Autodesk Inventor part; units mm, degrees
ref_plane "Work Plane1" through (29, 0, 0) normal (0, -1, 0) x (1, 0, 0)
ref_plane "YZ Plane" through (0, 0, 0) normal (1, 0, 0) x (0, 1, 0)
ref_plane "XZ Plane" through (0, 0, 0) normal (0, 1, 0) x (-1, 0, 0)
sketch "Sketch1" plane through (0, 0, 0) normal (0, 0, 1) x (1, 0, 0)
  line L0 (-0.9567, 0) -> (11.1125, 0)
  line L1 (11.1125, 0) -> (11.1125, 1.7526)
  line L2 (11.1125, 1.7526) -> (1.9847, 1.7526)
  line L3 (1.9847, 1.7526) -> (0.0001, 1.7526)
  line L4 (0.0001, 1.7526) -> (0, 1.7526)
  line L5 (0, 1.7526) -> (0, 2.8702)
  line L6 (0, 2.8702) -> (-3.5052, 2.8702)
  line L7 (-3.5052, 2.8702) -> (-3.5052, 1.5985)
  line L8 (-3.5052, 1.5985) -> (-1.8796, 1.5985)
  line L9 (-1.8796, 1.5985) -> (-0.9567, 0)
  line L10 (-6.4287, 0) -> (14.036, 0)
  line L11 (0, -0.574) -> (0, 3.4442)
  line L12 (1.9847, 1.7526) -> (0, 1.7526) construction
  dimension "d1" = 9.1278
  dimension "d2" = 1.9846
  dimension "d3" = 3.5052
  dimension "d4" = 1.6256
  dimension "d5" = 60
  dimension "d6" = 3.5052
  dimension "d7" = 3.5052
  dimension "d8" = 3.1969
  dimension "d9" = 5.7404
  dimension "d26" = 11.1125
revolve "Body" add sketch "Sketch1" angle 360 about axis through (-0.9567, 0, 0) along (1, 0, 0)
sketch "Sketch2" plane through (-3.5052, 0, 0) normal (-1, 0, 0) x (0, 0, 1)
  circle A0 centre (0, 0) radius 1.5985
  line L0 (0, -4.0183) -> (0, 4.0183)
  line L1 (-4.0183, 0) -> (4.0183, 0)
  line L2 (1.5985, 0) -> (0.7992, -1.3843)
  line L3 (0.7992, -1.3843) -> (-0.7992, -1.3843)
  line L4 (-0.7992, -1.3843) -> (-1.5985, 0)
  line L5 (-1.5985, 0) -> (-0.7992, 1.3843)
  line L6 (-0.7992, 1.3843) -> (0.7992, 1.3843)
  line L7 (0.7992, 1.3843) -> (1.5985, 0)
extrude "Slot" add sketch "Sketch2" against normal up to next contours L7 A0 | A0 L2 | L6 L0 A0 | A0 L0 L3 | L0 L6 A0 | A0 L3 L0 | L4 A0 | A0 L5
fillet "Fillet1" radius 0.3302 1 edges at (-3.5052, -2.8702, 0)
thread "Thread"
chamfer "Chamfer1" distance 0.4724 distance2 0.4724 1 edges at (11.1125, -1.7526, 0) measured on face at (11.1125, -0.5672, -0.1398)
ref_plane "Work Plane1" through (29, 0, 0) normal (0, -1, 0) x (1, 0, 0)
fillet "Fillet2" radius 0.127 1 edges at (0.0001, -1.7526, 0)
equation "\"d1\" = GEL"
equation "\"d3\" = KOH"
equation "\"d4\" = INTI"
equation "\"d6\" = GD"
equation "\"d7\" = BDM"
equation "\"d8\" = 1.1547 * SW"
equation "\"d9\" = KOD"
equation "\"d26\" = NLG"
equation "\"d30\" = R"
equation "\"d17\" = RR"
equation "\"d13\" = GEL"
equation "\"d15\" = -0.5 * SPD + 0.5 * GD"
equation "\"d16\" = GUL"
equation "\"GD\" = 3.5052"
equation "\"NLG\" = 11.1125"
equation "\"GEL\" = 9.1278"
equation "\"KOD\" = 5.7404"
equation "\"KOH\" = 3.5052"
equation "\"INTI\" = 1.6256"
equation "\"GAL\" = 1.9845"
equation "\"GUL\" = 0.47244"
equation "\"BDM\" = 3.5052"
equation "\"SW\" = 2.7686"
equation "\"RR\" = 0.3302"
equation "\"SPD\" = 2.56032"
equation "\"R\" = 0.127"
equation "\"PHH\" = 0.127"
equation "\"GD1\" = SPD"
equation "\"THREADDIA\" = 3.5052"
equation "\"FAWI\" = 45deg"
equation "\"KOH1\" = 3.1496"
equation "\"NND\" = 3.5052"
equation "\"TOA\" = 30deg"
equation "\"E0\" = 1.155 * SW"
properties part number "ANSI B18.3 - No. 6 - 32 UNC - 7/16 HS HCS" material "Steel, Mild"
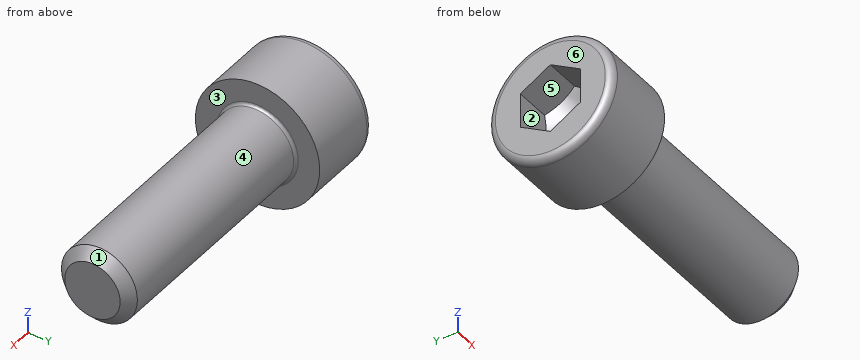
CAD build for the part. Positions are in the model's coordinates, mm. Face numbers are marked on the shaded views. A direction names the side the tool comes from. Coordinates: 2 decimals unless noted, no trailing zeros. Write each loop counter-clockwise with the first axis right and the second up, starting at its lowest first coordinate (ties: lowest second). Pieces come first, ordered by that corner, then holes. Notation, with made-up numbers: M 23,70 L 64,70 A23 cw 64,82 Z; hole C 79,82.25 d8. An arc over 180 degrees is marked long. Answer as a JSON object with one key per item and string values. Group by question number.
1) Mould opens along Y. For the marked faces 1, 2 and 3 say: +Y half, -Y half, draft (parallel to the pull), parting line (faces both ways), or undercut.
2) Pin check, flat tips, straight feed: pin 1 Ø1 at (x, z) = (2.5, -0.5) entering from -Y; pin 2 Ø3 at (x, z) = (-2, 0.5) entering from -Y. Stop position of each tip, or through.
3) Tool access for the marked faces 4, 5 and 6: list every direction of +Z, -Z, +X, -X, +Y, -Y with a clear straight run to the whole face (end or side of a thin tool).
4) Saw through at A-A (x = 6.5). Write the cut outline in (y, z), plus the area to 3 significant figures.
5) Saw through at B-B (x = -0.25). Write the cut outline in (y, z), plus the area to 3 significant figures.
6) Wall check: line 1 (X direction, y = 0.85, z = -2.2); line 2 (Z direction, x = 2.5, y = 0.05); line 3 (Y direction, x = -2.5, z = -1.8). Give the ranges that are in metal, low to high. Write a range as from..to.
Values follow:
{
 "1": {"face 1": "parting line", "face 2": "undercut", "face 3": "draft"},
 "2": {"pin 1": "stops at y = -1.75", "pin 2": "stops at y = -2.87"},
 "3": {"face 4": "+X", "face 5": "-X", "face 6": "+Z, -Z, -X, +Y, -Y"},
 "4": {"outline": "C 0,0 d3.51", "area": "9.65 mm2"},
 "5": {"outline": "C 0,0 d5.74", "area": "25.9 mm2"},
 "6": {"line 1": "x = -3.51..0", "line 2": "z = -1.75..1.75", "line 3": "y = -2.24..2.24"}
}
